Verification items for the finished model (mm, model axes). Round coordinates to 2 decimals unless told otherwise and drop trailing zeros. Order: outer loops, then holes, each group sorted by start corner. A loop starts at its lowest first (then second) coordinate and runs counter-clockwise, first axis right, second up. Notation, with made-up numbers: M 84.25,43.5 L 124.25,43.5 A16 cw 124.25,51.5 Z; hole C -6.5,-8.75 d1. An arc over 180 degrees is marked long. Use one line per item in the form item = value. Start each with the question number.
Item 1: Thickness scan on probe 1 along Z at (x, y) = (24.5, 47); probe 2 along Y at (x, z) = (277.5, 3.5); probe 3 along X at (y, z) = (48.5, 2.5). Record the ranges inside material, lowest first. Write a range as [from, to].
Item 2: Cross-section at B-B on y = 25. Enter the section's corners in (x, z), then the cut area to 3 significant figures.
Item 3: Go/stop test with flat-tipped pins: pin 1 Ø0.8 at (y, z) = (49, 0.5) entering from -X; pin 2 Ø6.5 at (x, y) = (11.5, 47) entering from +Z; pin 3 Ø1.5 at (y, z) = (48, 6) entering from -X. Record where each tip stops, or that it passes through.
Item 4: Cross-section at A-A on z = 5.75. Enter the section's corners in (x, y), then the cut area to 3 significant figures.
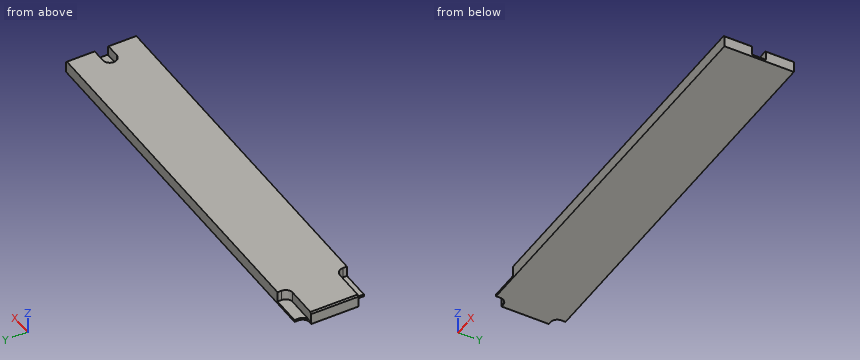
from build123d import *

# Parameters (mm, degrees)
BASE_EXTRUDE_DEPTH = 9
CUT_EXTRUDE1_DEPTH = 7.5
CHAMFER1_SIZE      = 1


with BuildPart() as part:
    # Sketch1 → Base-Extrude (new body)
    with BuildSketch(Plane.XY):
        with BuildLine():
            Line((7, 0), (290, 0))
            Line((290, 0), (290, 50))
            Line((290, 50), (7, 50))
            Line((7, 50), (7, 47))
            ThreePointArc((7, 47), (5.535533906, 43.464466094), (2, 42))
            Line((2, 42), (0, 42))
            Line((0, 42), (0, 8))
            Line((0, 8), (2, 8))
            ThreePointArc((2, 8), (5.535533906, 6.535533906), (7, 3))
            Line((7, 3), (7, 0))
        make_face()
    extrude(amount=BASE_EXTRUDE_DEPTH)

    # Sketch2 → Cut-Extrude1 (cut)
    with BuildSketch(Plane.XY.offset(9)):
        with BuildLine():
            Line((2, 8), (23, 8))
            ThreePointArc((23, 8), (26.535533906, 6.535533906), (28, 3))
            Line((28, 3), (28, 0))
            Line((28, 0), (2, 0))
            Line((2, 0), (2, 8))
        make_face()
        with BuildLine():
            Line((279, 30), (290, 30))
            Line((290, 30), (290, 20))
            Line((290, 20), (279, 20))
            ThreePointArc((279, 20), (274, 25), (279, 30))
        make_face()
        with BuildLine():
            Line((28, 47), (28, 50))
            Line((28, 50), (2, 50))
            Line((2, 50), (2, 42))
            Line((2, 42), (23, 42))
            ThreePointArc((23, 42), (26.535533906, 43.464466094), (28, 47))
        make_face()
    extrude(amount=-CUT_EXTRUDE1_DEPTH, mode=Mode.SUBTRACT)

    # Chamfer1
    chamfer1_edges = [part.edges().sort_by_distance(p)[0] for p in [
        (0, 25, 9),
        (290, 40, 9),
        (290, 10, 9),
    ]]
    chamfer(chamfer1_edges, length=CHAMFER1_SIZE)


solid = part.part
Output values:
q1.probe_1 = [0, 1.5]
q1.probe_2 = [0, 20.23], [29.77, 50]
q1.probe_3 = [28, 290]
q2.outline = M 0,0 L 290,0 L 290,1.5 L 274,1.5 L 274,9 L 1,9 L 0,8 Z
q2.area = 2,490 mm2
q3.pin_1 = 7
q3.pin_2 = 1.5
q3.pin_3 = 28
q4.outline = M 0,8 L 23,8 A5 cw 28,3 L 28,0 L 290,0 L 290,20 L 279,20 A5 cw 279,30 L 290,30 L 290,50 L 28,50 L 28,47 A5 cw 23,42 L 0,42 Z
q4.area = 13,900 mm2
